from build123d import *

# Parameters (mm, degrees)
SKETCH1_R           = 3
BOSS_EXTRUDE1_DEPTH = 3
SKETCH2_W           = 28
SKETCH2_H           = 5
CUT_EXTRUDE1_DEPTH  = 79.545892535
CUT_EXTRUDE2_DEPTH  = 79.545892535


with BuildPart() as part:
    # Sketch1 → Boss-Extrude1 (new body)
    with BuildSketch(Plane(origin=(0, 0, 0), x_dir=(1, 0, 0), z_dir=(0, 1, 0))):
        with BuildLine():
            Line((55.872458647, -40.12463695), (55.872458647, 39.87536305))
            ThreePointArc((55.872458647, 39.87536305), (51.479060365, 50.481964768), (40.872458647, 54.87536305))
            Line((40.872458647, 54.87536305), (-39.127541353, 54.87536305))
            ThreePointArc((-39.127541353, 54.87536305), (-49.734143071, 50.481964768), (-54.127541353, 39.87536305))
            Line((-54.127541353, 39.87536305), (-54.127541353, -40.12463695))
            ThreePointArc((-54.127541353, -40.12463695), (-49.734143071, -50.731238667), (-39.127541353, -55.12463695))
            Line((-39.127541353, -55.12463695), (40.872458647, -55.12463695))
            ThreePointArc((40.872458647, -55.12463695), (51.479060365, -50.731238667), (55.872458647, -40.12463695))
        make_face()
        with Locations(Location((48.872458647, 32.87536305, 0), (0, 0, 270))):
            Circle(SKETCH1_R, mode=Mode.SUBTRACT)
        with Locations(Location((-47.127541353, -33.12463695, 0), (0, 0, 270))):
            Circle(SKETCH1_R, mode=Mode.SUBTRACT)
        with Locations(Location((-32.127541353, -48.12463695, 0), (0, 0, 270))):
            Circle(SKETCH1_R, mode=Mode.SUBTRACT)
        with Locations(Location((33.872458647, -48.12463695, 0), (0, 0, 270))):
            Circle(SKETCH1_R, mode=Mode.SUBTRACT)
        with Locations(Location((48.872458647, -33.12463695, 0), (0, 0, 270))):
            Circle(SKETCH1_R, mode=Mode.SUBTRACT)
        with Locations(Location((33.872458647, 47.87536305, 0), (0, 0, 270))):
            Circle(SKETCH1_R, mode=Mode.SUBTRACT)
        with Locations(Location((-32.127541353, 47.87536305, 0), (0, 0, 270))):
            Circle(SKETCH1_R, mode=Mode.SUBTRACT)
        with Locations(Location((-47.127541353, 32.87536305, 0), (0, 0, 270))):
            Circle(SKETCH1_R, mode=Mode.SUBTRACT)
    extrude(amount=BOSS_EXTRUDE1_DEPTH)

    # Sketch2 → Cut-Extrude1 (cut, through all)
    with BuildSketch(Plane(origin=(0, 3, 0), x_dir=(1, 0, 0), z_dir=(0, 1, 0))):
        with Locations((0.872458647, -40.12463695)):
            Rectangle(SKETCH2_W, SKETCH2_H)
    extrude(amount=-CUT_EXTRUDE1_DEPTH, mode=Mode.SUBTRACT)

    # Sketch3 → Cut-Extrude2 (cut, through all)
    with BuildSketch(Plane(origin=(0, 3, 0), x_dir=(1, 0, 0), z_dir=(0, 1, 0))):
        Polygon((40, -34.343145751), (5.656854249, 0), (40, 34.343145751), align=None)
        Polygon((34.343145751, -40), (18.872458647, -40), (18.872458647, -39.281491199), (26.248547798, -31.905402048), align=None)
        Polygon((34.343145751, 40), (-34.343145751, 40), (0, 5.656854249), align=None)
        Polygon((-40, -34.343145751), (-40, 34.343145751), (-5.656854249, 0), align=None)
        Polygon((0, -5.656854249), (-19.719234902, -25.376089151), (-11.470687104, -33.62463695), (13.215604397, -33.62463695), (20.591693549, -26.248547798), align=None)
        Polygon((-17.127541353, -39.281491199), (-17.127541353, -40), (-34.343145751, -40), (-25.376089151, -31.032943401), align=None)
    extrude(amount=-CUT_EXTRUDE2_DEPTH, mode=Mode.SUBTRACT)


solid = part.part
Work out the finished part from the listing and answer in its coordinate system (mm). A direction names the side the tool comes from. Coordinates: 2 decimals unless noted, no trailing zeros. Write each loop counter-clockwise with the first axis right and the second up, starting at its lowest first coordinate (ties: lowest second). Pieces come first, ordered by that corner, then holes. Notation, with made-up numbers: M 19.5,83 L 74.5,83 A25 cw 74.5,102 Z; hole C 20,67 d10. An arc over 180 degrees is marked long. Answer as CSV lines item,"result". Start each with the question number.
Item 1: Consider L1, parallel to X at y = 1.2, z = -8; L2, parallel to X at y = 0.55, z = 37.5; L3, parallel to X at y = 0.95, z = 27.5. Determine where each line is inside the solid, lowest interval first.
Item 2: Section C-C on z = 3 is taken. Write down the section's boundary in (x, y).
Item 3: Section B-B on x = 27.5 is taken. Write down the section's boundary in (y, z).
Item 4: Section D-D on x = 10.5 is taken. Write down the section's boundary in (y, z).
Item 5: A flat-ended cylindrical pin translates along its axis: P1, Ø3.5, axis at x = 33.87, z = -47.88, coming from the -Y side (3 decimals). Find the tip coordinate at first contact, or state that the pin passes through.
Item 6: Section A-A on z = 22.5 is taken. Write down the section's boundary in (x, y), and give its area (3 significant figures).
Item 7: A tool of negligible diameter and unlimited length cuts with its end or side. For faces 4 (the face through (-49.617, 1.479, -50.598)), 5 (the face through (40, 2, 0)), from which of +Z, -Z, +X, -X, +Y, -Y can it reach the whole face along a straight path? Write none if from no direction.
Item 8: Determine the mould class of faces 1 (the face through (-49.85, 1.479, 50.614)), 2 (the face through (0, 3, -1)), 3 (the face through (-15.653, 1.521, 29.443)) for opening direction Z: released by +Z, released by -Z, zero draft, split by the parting line, or undercut.
Checks:
1,L1,"x = -54.13 to -40, -13.66 to -2.34, 2.34 to 13.66, 40 to 55.87"
1,L2,"x = -54.13 to -31.84, -18.91 to 20.65, 31.84 to 55.87"
1,L3,"x = -54.13 to -40, -33.16 to -17.6, 19.34 to 33.16, 40 to 55.87"
2,outline,"M -54.13,0 L -40,0 L -40,3 L -54.13,3 Z; M -8.66,0 L 8.66,0 L 8.66,3 L -8.66,3 Z; M 40,0 L 55.87,0 L 55.87,3 L 40,3 Z"
3,outline,"M 0,-54.88 L 3,-54.88 L 3,-40 L 0,-40 Z; M 0,-33.16 L 3,-33.16 L 3,-21.84 L 0,-21.84 Z; M 0,21.84 L 3,21.84 L 3,33.16 L 0,33.16 Z; M 0,40 L 3,40 L 3,55.12 L 0,55.12 Z"
4,outline,"M 0,-54.88 L 3,-54.88 L 3,-40 L 0,-40 Z; M 0,-16.16 L 3,-16.16 L 3,-4.84 L 0,-4.84 Z; M 0,4.84 L 3,4.84 L 3,16.16 L 0,16.16 Z; M 0,33.62 L 3,33.62 L 3,37.62 L 0,37.62 Z; M 0,42.62 L 3,42.62 L 3,55.12 L 0,55.12 Z"
5,P1,"passes through"
6,outline,"M -54.13,0 L -40,0 L -40,3 L -54.13,3 Z; M -28.16,0 L -16.84,0 L -16.84,3 L -28.16,3 Z; M 16.84,0 L 28.16,0 L 28.16,3 L 16.84,3 Z; M 40,0 L 55.87,0 L 55.87,3 L 40,3 Z"
6,area,"158 mm²"
7,face 4,"-Z, -X, +Y, -Y"
7,face 5,"+Y, -Y"
8,face 1,"released by +Z"
8,face 2,"zero draft"
8,face 3,"undercut"
